Could you check a few things on this model? Use its own coordinates, in mm. A direction names the side the tool comes from. Round coordinates to 2 decimals unless told otherwise and drop trailing zeros. Write each loop counter-clockwise with the first axis right and the second up, starting at its lowest first coordinate (ties: lowest second). Pieces come first, ordered by that corner, then holes. Notation, with made-up numbers: M 6,29 L 25,29 A27 cw 25,68 Z; hole C 54,38.5 d1. An arc over 180 degrees is marked long. One line per question, with ' | ' between items. Start each with the question number.
```python
from build123d import *

# Parameters (mm, degrees)
SKETCH1_R           = 2.9
BOSS_EXTRUDE1_DEPTH = 5
BOSS_EXTRUDE2_DEPTH = 13
SKETCH4_R           = 2.9
BOSS_EXTRUDE3_DEPTH = 3
BOSS_EXTRUDE4_DEPTH = 21
SKETCH7_W           = 57.588234794
SKETCH7_H           = 15
SKETCH7_R           = 2
BOSS_EXTRUDE6_DEPTH = 5
SKETCH9_W           = 10.98683059
SKETCH9_H           = 21
SKETCH9_R           = 2
BOSS_EXTRUDE7_DEPTH = 5


with BuildPart() as part:
    # Sketch1 → Boss-Extrude1 (new body)
    with BuildSketch(Plane(origin=(0, 0, 0), x_dir=(1, 0, 0), z_dir=(0, 1, 0))):
        with BuildLine():
            Line((62.90038715, 19.069123632), (73.88721774, 26.399609553))
            ThreePointArc((73.88721774, 26.399609553), (77.156269753, 33.244214317), (73.88721774, 40.088819081))
            Line((73.88721774, 40.088819081), (62.90038715, 47.419305002))
            ThreePointArc((62.90038715, 47.419305002), (58.150415973, 50.856886947), (53.675790472, 54.645939921))
            ThreePointArc((53.675790472, 54.645939921), (34.106269753, 62.244214317), (14.536749034, 54.645939921))
            ThreePointArc((14.536749034, 54.645939921), (10.062123533, 50.856886947), (5.312152356, 47.419305002))
            Line((5.312152356, 47.419305002), (-5.674678234, 40.088819081))
            ThreePointArc((-5.674678234, 40.088819081), (-8.943730247, 33.244214317), (-5.674678234, 26.399609553))
            Line((-5.674678234, 26.399609553), (5.312152356, 19.069123632))
            ThreePointArc((5.312152356, 19.069123632), (10.062123533, 15.631541687), (14.536749034, 11.842488713))
            ThreePointArc((14.536749034, 11.842488713), (34.106269753, 4.244214317), (53.675790472, 11.842488713))
            ThreePointArc((53.675790472, 11.842488713), (58.150415973, 15.631541687), (62.90038715, 19.069123632))
        make_face()
        with Locations((68.356269753, 33.244214317)):
            Circle(SKETCH1_R, mode=Mode.SUBTRACT)
        with Locations((-0.143730247, 33.244214317)):
            Circle(SKETCH1_R, mode=Mode.SUBTRACT)
    extrude(amount=BOSS_EXTRUDE1_DEPTH)

    # Sketch3 → Boss-Extrude2 (add)
    with BuildSketch(Plane(origin=(0, 5, 0), x_dir=(1, 0, 0), z_dir=(0, 1, 0))):
        with BuildLine():
            Line((62.90038715, 19.069123632), (73.88721774, 26.399609553))
            ThreePointArc((73.88721774, 26.399609553), (77.011551697, 31.654845113), (75.9581291, 37.677242003))
            Line((75.9581291, 37.677242003), (74.027243913, 37.677242003))
            Line((74.027243913, 37.677242003), (74.156269753, 33.244214317))
            ThreePointArc((74.156269753, 33.244214317), (73.616142187, 30.800090348), (72.096358727, 28.811186631))
            Line((72.096358727, 28.811186631), (61.235353843, 21.564652451))
            ThreePointArc((61.235353843, 21.564652451), (56.300318854, 17.993138742), (51.651357294, 14.056460327))
            ThreePointArc((51.651357294, 14.056460327), (34.106269753, 7.244214317), (16.561182212, 14.056460327))
            ThreePointArc((16.561182212, 14.056460327), (11.912220652, 17.993138742), (6.977185663, 21.564652451))
            Line((6.977185663, 21.564652451), (-3.883819221, 28.811186631))
            ThreePointArc((-3.883819221, 28.811186631), (-5.403602681, 30.800090348), (-5.943730247, 33.244214317))
            Line((-5.943730247, 33.244214317), (-5.814704408, 37.677242003))
            Line((-5.814704408, 37.677242003), (-7.745589594, 37.677242003))
            ThreePointArc((-7.745589594, 37.677242003), (-8.799012191, 31.654845113), (-5.674678234, 26.399609553))
            Line((-5.674678234, 26.399609553), (5.312152356, 19.069123632))
            ThreePointArc((5.312152356, 19.069123632), (10.062123533, 15.631541687), (14.536749034, 11.842488713))
            ThreePointArc((14.536749034, 11.842488713), (34.106269753, 4.244214317), (53.675790472, 11.842488713))
            ThreePointArc((53.675790472, 11.842488713), (58.150415973, 15.631541687), (62.90038715, 19.069123632))
        make_face()
    extrude(amount=BOSS_EXTRUDE2_DEPTH)

    # Sketch4 → Boss-Extrude3 (add)
    with BuildSketch(Plane(origin=(0, 18, 0), x_dir=(1, 0, 0), z_dir=(0, 1, 0))):
        with BuildLine():
            Line((3.616180779, 37.677242003), (-7.745589594, 37.677242003))
            ThreePointArc((-7.745589594, 37.677242003), (-8.799012191, 31.654845113), (-5.674678234, 26.399609553))
            Line((-5.674678234, 26.399609553), (5.312152356, 19.069123632))
            ThreePointArc((5.312152356, 19.069123632), (10.062123533, 15.631541687), (14.536749034, 11.842488713))
            ThreePointArc((14.536749034, 11.842488713), (34.106269753, 4.244214317), (53.675790472, 11.842488713))
            ThreePointArc((53.675790472, 11.842488713), (58.150415973, 15.631541687), (62.90038715, 19.069123632))
            Line((62.90038715, 19.069123632), (73.88721774, 26.399609553))
            ThreePointArc((73.88721774, 26.399609553), (77.011551697, 31.654845113), (75.9581291, 37.677242003))
            Line((75.9581291, 37.677242003), (64.596358727, 37.677242003))
            Line((64.596358727, 37.677242003), (61.235353843, 21.564652451))
            ThreePointArc((61.235353843, 21.564652451), (56.300318854, 17.993138742), (51.651357294, 14.056460327))
            ThreePointArc((51.651357294, 14.056460327), (34.106269753, 7.244214317), (16.561182212, 14.056460327))
            ThreePointArc((16.561182212, 14.056460327), (11.912220652, 17.993138742), (6.977185663, 21.564652451))
            Line((6.977185663, 21.564652451), (3.616180779, 37.677242003))
        make_face()
        with Locations((-0.143730247, 33.244214317)):
            Circle(SKETCH4_R, mode=Mode.SUBTRACT)
        with Locations((68.356269753, 33.244214317)):
            Circle(SKETCH4_R, mode=Mode.SUBTRACT)
    extrude(amount=BOSS_EXTRUDE3_DEPTH)

    # Sketch5 → Boss-Extrude4 (add)
    with BuildSketch(Plane.XZ):
        with BuildLine():
            Line((62.90038715, -19.069123632), (62.90038715, 5.755785683))
            Line((62.90038715, 5.755785683), (5.312152356, 5.755785683))
            Line((5.312152356, 5.755785683), (5.312152356, -19.069123632))
            ThreePointArc((5.312152356, -19.069123632), (10.062123533, -15.631541687), (14.536749034, -11.842488713))
            ThreePointArc((14.536749034, -11.842488713), (34.106269753, -4.244214317), (53.675790472, -11.842488713))
            ThreePointArc((53.675790472, -11.842488713), (58.150415973, -15.631541687), (62.90038715, -19.069123632))
        make_face()
    extrude(amount=-BOSS_EXTRUDE4_DEPTH)

    # Sketch7 → Boss-Extrude6 (add)
    with BuildSketch(Plane.XY.offset(5.755785683)):
        with Locations((34.106269753, 28.5)):
            Rectangle(SKETCH7_W, SKETCH7_H)
        with Locations((34.106269753, 28.5)):
            Circle(SKETCH7_R, mode=Mode.SUBTRACT)
    extrude(amount=-BOSS_EXTRUDE6_DEPTH)

    # Sketch9 → Boss-Extrude7 (add)
    with BuildSketch(Plane.XY.offset(5.755785683)):
        with Locations((68.393802445, 10.5)):
            Rectangle(SKETCH9_W, SKETCH9_H)
        with Locations((68.393802445, 10.5)):
            Circle(SKETCH9_R, mode=Mode.SUBTRACT)
        with Locations((-0.181262939, 10.5)):
            Rectangle(SKETCH9_W, SKETCH9_H)
        with Locations((-0.181262939, 10.5)):
            Circle(SKETCH9_R, mode=Mode.SUBTRACT)
    extrude(amount=-BOSS_EXTRUDE7_DEPTH)


solid = part.part
```
1. Suppose I cut it at D-D (z = -11.5). Write out the boundary of the cut face in (x, y), and give its area (3 significant figures).
2. If we mould it in two halves opening along Z, with no side actions, what happens to faces 1 (the face through (34, 36, 3)), 2 (the face through (-2.445, 2.465, -31.48)), 3 (the face through (34.376, 12.888, -7.246))? For each: released by +Z, released by -Z, zero draft, split by the parting line, or undercut.
3. I need wall thicknesses on line 1 along Y through (x, z) = (64, -32); line 2 along Y through (x, z) = (21.5, -18.5); line 3 along X through (y, z) = (3.5, -31). Which ranges of each line are inside material? Lowest first, please. Write a range as from..to.
4. Suppose I cut it at C-C (z = -20). Write out the boundary of the cut face in (x, y).
5. Which directions (+Z, -Z, +X, -X, +Y, -Y) give clear straight access to the entire face, cutting with the end or side of a thin tool? Please do faces 4 (the face through (73.887, 10, 3)), 5 (the face through (0, 21, 3)), 6 (the face through (-0.442, 12.483, 3.291)).
6. Suppose I cut it at A-A (y = 28.5). Write out the boundary of the cut face in (x, z).
7. Suppose I cut it at B-B (y = 10.5). Count the separate pieces of the cut face and the enclosed holes in it, and give its area (3 significant figures).
8. I'm going to push flat-ended pins straight in: P1, Ø1, axis at y = 10.5, z = -16.5, coming from the -X side; P2, Ø7.5, axis at x = -0.14, z = -33.24, coming from the +Y side; P3, Ø4, axis at y = 6, z = -45, coming from the +X side. Where does each tip first touch, or does it pass through?
Computed:
1) outline: M 5.31,0 L 62.9,0 L 62.9,21 L 48.36,21 L 48.36,5 L 19.85,5 L 19.85,21 L 5.31,21 Z | area: 753 mm²
2) face 1: zero draft | face 2: undercut | face 3: released by -Z
3) line 1: y = 0..5, 18..21 | line 2: y = 0..5 | line 3: x = -8.65..-1.98, 1.69..66.52, 70.19..76.87
4) outline: M 3.92,0 L 64.3,0 L 64.3,21 L 58.98,21 L 58.98,5 L 9.24,5 L 9.24,21 L 3.92,21 Z
5) face 4: +Z, +X, +Y, -Y | face 5: +Z, -Z, -X, +Y | face 6: +Z
6) outline: M 5.31,0.76 L 32.11,0.76 L 32.11,5.76 L 5.31,5.76 Z; M 36.11,0.76 L 62.9,0.76 L 62.9,5.76 L 36.11,5.76 Z
7) separate pieces: 3 | enclosed holes: 0 | area: 1,280 mm²
8) P1: stops at x = 5.31 | P2: stops at y = 21 | P3: stops at x = 69.12
